Autodesk Inventor part; units mm, degrees
ref_plane "YZ Plane" through (0, 0, 0) normal (1, 0, 0) x (0, 1, 0)
ref_plane "XZ Plane" through (0, 0, 0) normal (0, 1, 0) x (-1, 0, 0)
ref_plane "XY Plane" through (0, 0, 0) normal (0, 0, 1) x (1, 0, 0)
sketch "Sketch1" plane through (0, 0, 0) normal (0, 1, 0) x (-1, 0, 0)
  circle A0 centre (0, 0) radius 350
  circle A1 centre (0, 0) radius 370
  line L0 (370, 0) -> (350, 0)
  line L1 (-370, 0) -> (-350, 0)
  line L2 (0, 0) -> (-350, 0) construction
  line L3 (0, 350) -> (0, 0) construction
  line L4 (0, 370) -> (0, 350)
  line L5 (-350, 0) -> (-370, 0)
  line L6 (-354, 7) -> (-366, 7)
  line L7 (-366, 7) -> (-363.4522, 0)
  line L8 (-354, 7) -> (-356.5478, 0)
  line L9 (-360, 0) -> (-360, 7) construction
  line L10 (-356.9749, 57.6407) -> (-350.9683, 87.0332)
  line L11 (-350.9683, 87.0332) -> (-347.8331, 86.3925)
  line L12 (-347.8331, 86.3925) -> (-353.8397, 57)
  line L13 (-353.8397, 57) -> (-356.9749, 57.6407)
  line L14 (-356.9749, 57.6407) -> (-347.8331, 86.3925) construction
  line L15 (-350.9683, 87.0332) -> (-353.8397, 57) construction
  circle A2 centre (0, 0) radius 360 construction
  line L16 (-7, -354) -> (0, -356.5478)
  line L17 (-7, -366) -> (0, -363.4522)
  line L18 (-7, -354) -> (-7, -366)
  line L19 (354, -7) -> (356.5478, 0)
  line L20 (366, -7) -> (363.4522, 0)
  line L21 (354, -7) -> (366, -7)
  line L22 (7, 354) -> (0, 356.5478)
  line L23 (7, 366) -> (0, 363.4522)
  line L24 (7, 354) -> (7, 366)
  line L25 (-337.9697, -128.5692) -> (-347.4641, -100.1112)
  line L26 (-334.9342, -127.5564) -> (-337.9697, -128.5692)
  line L27 (-344.4286, -99.0984) -> (-334.9342, -127.5564)
  line L28 (-347.4641, -100.1112) -> (-344.4286, -99.0984)
  line L29 (-228.4058, -280.329) -> (-250.8572, -260.4309)
  line L30 (-226.2833, -277.9342) -> (-228.4058, -280.329)
  line L31 (-248.7347, -258.0361) -> (-226.2833, -277.9342)
  line L32 (-250.8572, -260.4309) -> (-248.7347, -258.0361)
  line L33 (-57.6407, -356.9749) -> (-87.0332, -350.9683)
  line L34 (-57, -353.8397) -> (-57.6407, -356.9749)
  line L35 (-86.3925, -347.8331) -> (-57, -353.8397)
  line L36 (-87.0332, -350.9683) -> (-86.3925, -347.8331)
  line L37 (128.5692, -337.9697) -> (100.1112, -347.4641)
  line L38 (127.5564, -334.9342) -> (128.5692, -337.9697)
  line L39 (99.0984, -344.4286) -> (127.5564, -334.9342)
  line L40 (100.1112, -347.4641) -> (99.0984, -344.4286)
  line L41 (280.329, -228.4058) -> (260.4309, -250.8572)
  line L42 (277.9342, -226.2833) -> (280.329, -228.4058)
  line L43 (258.0361, -248.7347) -> (277.9342, -226.2833)
  line L44 (260.4309, -250.8572) -> (258.0361, -248.7347)
  line L45 (356.9749, -57.6407) -> (350.9683, -87.0332)
  line L46 (353.8397, -57) -> (356.9749, -57.6407)
  line L47 (347.8331, -86.3925) -> (353.8397, -57)
  line L48 (350.9683, -87.0332) -> (347.8331, -86.3925)
  line L49 (337.9697, 128.5692) -> (347.4641, 100.1112)
  line L50 (334.9342, 127.5564) -> (337.9697, 128.5692)
  line L51 (344.4286, 99.0984) -> (334.9342, 127.5564)
  line L52 (347.4641, 100.1112) -> (344.4286, 99.0984)
  line L53 (228.4058, 280.329) -> (250.8572, 260.4309)
  line L54 (226.2833, 277.9342) -> (228.4058, 280.329)
  line L55 (248.7347, 258.0361) -> (226.2833, 277.9342)
  line L56 (250.8572, 260.4309) -> (248.7347, 258.0361)
  line L57 (57.6407, 356.9749) -> (87.0332, 350.9683)
  line L58 (57, 353.8397) -> (57.6407, 356.9749)
  line L59 (86.3925, 347.8331) -> (57, 353.8397)
  line L60 (87.0332, 350.9683) -> (86.3925, 347.8331)
  line L61 (-128.5692, 337.9697) -> (-100.1112, 347.4641)
  line L62 (-127.5564, 334.9342) -> (-128.5692, 337.9697)
  line L63 (-99.0984, 344.4286) -> (-127.5564, 334.9342)
  line L64 (-100.1112, 347.4641) -> (-99.0984, 344.4286)
  line L65 (-280.329, 228.4058) -> (-260.4309, 250.8572)
  line L66 (-277.9342, 226.2833) -> (-280.329, 228.4058)
  line L67 (-258.0361, 248.7347) -> (-277.9342, 226.2833)
  line L68 (-260.4309, 250.8572) -> (-258.0361, 248.7347)
  point P0 (360, 0)
  point P1 (-360, 0)
  point P2 (-352.404, 72.0166)
  point P3 (-68.8261, 353.3595)
  point P4 (-355.4073, 57.3204)
  point P5 (-349.4007, 86.7129)
  point P6 (-7, -360)
  point P7 (360, -7)
  point P8 (7, 360)
  point P9 (-336.452, -128.0628)
  point P10 (-345.9464, -99.6048)
  point P11 (-227.3446, -279.1316)
  point P12 (-249.7959, -259.2335)
  point P13 (-57.3204, -355.4073)
  point P14 (-86.7129, -349.4007)
  point P15 (128.0628, -336.452)
  point P16 (99.6048, -345.9464)
  point P17 (279.1316, -227.3446)
  point P18 (259.2335, -249.7959)
  point P19 (355.4073, -57.3204)
  point P20 (349.4007, -86.7129)
  point P21 (336.452, 128.0628)
  point P22 (345.9464, 99.6048)
  point P23 (227.3446, 279.1316)
  point P24 (249.7959, 259.2335)
  point P25 (57.3204, 355.4073)
  point P26 (86.7129, 349.4007)
  point P27 (-128.0628, 336.452)
  point P28 (-99.6048, 345.9464)
  point P29 (-279.1316, 227.3446)
  point P30 (-259.2335, 249.7959)
  point P31 (0, 356.5478)
  point P32 (0, 363.4522)
  dimension "d0" = 700
  dimension "d1" = 740
  dimension "d4" = 90
  dimension "d5" = 7
  dimension "d6" = 70
  dimension "d8" = 12
  dimension "d13" = 3.2
  dimension "d14" = 30
  dimension "d15" = 50
  dimension "d20" = 720
  dimension "d23" = 360
  dimension "d27" = 360
extrude "Extrusion1" add sketch "Sketch1" along normal blind 3 contours A0 L1 L8 L6 L7 A1 L4 | L4 L23 L24 L22
properties part number "R70_CM_CIRCULO"
CAD build for the part. Positions are in the model's coordinates, mm. A direction names the side the tool comes from. Round coordinates to 2 decimals unless told otherwise and drop trailing zeros. Order: outer loops, then holes, each group sorted by start corner. A loop starts at its lowest first (then second) coordinate and runs counter-clockwise, first axis right, second up. Notation, with made-up numbers: M 17,-13 L 68,-13 A20 cw 68,3 Z; hole C 7.25,4.25 d10. An arc over 180 degrees is marked long. Use one line per item in the form item = value.
Q1. Saw through at A-A on y = 1.45. Give the cut face in (x, z), then the cut area to 3 significant figures.
Recorded:
outline = M -7,354 L 0,356.55 L 0,350 A350 cw 350,0 L 356.55,0 L 354,7 L 366,7 L 363.45,0 L 370,0 A370 ccw 0,370 L 0,363.45 L -7,366 Z; hole M 99.1,344.43 L 127.56,334.93 L 128.57,337.97 L 100.11,347.46 Z; hole M 258.04,248.73 L 277.93,226.28 L 280.33,228.41 L 260.43,250.86 Z; hole M 347.83,86.39 L 353.84,57 L 356.97,57.64 L 350.97,87.03 Z
area = 11,000 mm^2
Q2. Two-plate mould, pull along X, no slides. Class faces 3 (the cylindrical face through (250.194, 1.479, 244.751)), 4 (the flat face through (267.846, 1.479, 237.666)), 5 (the flat face through (114.54, 1.48, 342.65)), 6 (the cylindrical face through (264.49, 1.48, 258.74)): +X half, -X half, draft (parallel to the pull), parting line (faces both ways), or undercut.
Recorded:
face_3 = -X half
face_4 = undercut
face_5 = undercut
face_6 = +X half
Q3. Saw through at C-C on x = 200.5. Give the cut face in (y, z), then the cut area to 3 significant figures.
Recorded:
outline = M 0,286.88 L 3,286.88 L 3,310.97 L 0,310.97 Z
area = 72.3 mm^2
Q4. Saw through at D-D on z = 40. Give the cut face in (x, y), then the cut area to 3 significant figures.
Recorded:
outline = M 347.71,0 L 367.83,0 L 367.83,3 L 347.71,3 Z
area = 60.4 mm^2
Q5. Saw through at B-B on z = 79. Give the cut face in (x, y), then the cut area to 3 significant figures.
Recorded:
outline = M 340.97,0 L 349.34,0 L 349.34,3 L 340.97,3 Z; M 352.61,0 L 361.47,0 L 361.47,3 L 352.61,3 Z
area = 51.7 mm^2
Q6. Probe L1, parallel to X at y = 2.6, z = 242.5; L2, parallel to Z at x = 266.5, y = 2.05; L3, parallel to Z at x = 171, y = 1.8. List the from-to ranges inside material, lowest first.
Recorded:
L1 = 252.38 to 263.56, 267.84 to 279.45
L2 = 226.89 to 239.18, 244.01 to 256.67
L3 = 305.38 to 328.11
Q7. Which spindle directions (+Z, -Z, +X, -X, +Y, -Y) get a long thin tool onto all of the face, cutting with end or side? Do faces 1 (the flat face through (270.519, 1.479, 239.474)), 2 (the flat face through (252, 0, 254)). Say none if no direction does.
Recorded:
face_1 = +Y, -Y
face_2 = +Z, -Z, +X, -X, -Y
Q8. Flat gauge pins, fed straight in: P1, Ø3, axis at x = 218, z = 271, coming from the +Y side (1 decimal); P2, Ø1.5, axis at x = 32.5, y = 1.5, coming from the +Z side. Where does each tip first touch, or does it go through?
Recorded:
P1 = through
P2 = 368.64
